Build history of the part. All positions in model axes, mm. A direction names the side the tool comes from. Give positions to 0.01 mm unless a question says otherwise; leave off trailing zeros. Order: outer loops, then holes, each group sorted by start corner. A loop starts at its lowest first (then second) coordinate and runs counter-clockwise, first axis right, second up. Notation, with made-up numbers: (-4, 19.5) -> (40, 19.5) arc R7 cw to (40, 25.5) -> close; hole circle Ø3 at (31, 7.25). An arc over 180 degrees is marked (long way). One line per question, with ' | ' between items. Start each with the question number.
(1) Cut at A-A (y = 241). Give the number of separate pieces and of enclosed holes in the cut face, then the cut area to 3 significant figures.
(2) Pin check, flat tips, straight feed: pin 1 Ø9.5 at (y, z) = (290, 16.5) entering from +X; pin 2 Ø2 at (x, y) = (-1077, -46) entering from +Z; pin 3 Ø9.5 at (x, z) = (-1638, 15) entering from +Y; pin 4 Ø2 at (y, z) = (271, 33.5) entering from +X. Stop position of each tip, or through.
(3) Which spindle directions (+Z, -Z, +X, -X, +Y, -Y) get a long thin tool onto all of the face, cutting with end or side? Do faces 1 (the face through (-2160.586, -325, 25)), 2 (the face through (0, 109, 25)), 3 (the face through (-1174, 155, 31.75)). Say none if no direction does.
(4) Cut at D-D (x = -989). Give the cut face in (y, z), then the cut area to 3 significant figures.
(5) Cut at B-B (x = -1476). Give the cut face in (y, z), then the cut area to 3 significant figures.
(6) Pull direction Y, two halves, no side cores. Call faces 4 (the face through (-1098, -116, 0)), 5 (the face through (-1163, 138.261, 38)), 6 (the face through (-1009, -296.136, 38)), 7 (the face through (-1097, -197, 31.75)): +Y half, -Y half, draft (parallel to the pull), parting line (faces both ways), or undercut.
(7) Drill centre lines: L1, parallel to Y at x = -1071, z = 34.5; L2, parallel to X at y = -323.5, z = 31 (3 decimals); L3, parallel to Y at x = -1812, z = 10. Where is each one in solid material? Low to high. Write a range as from..to.
from build123d import *

# Parameters (mm, degrees)
F2_DEPTH = 31.75
F1_W     = 2314.862013
F1_H     = 57.149999
F1_W_2   = 2314.703077
F1_H_2   = 57.15
F3_DEPTH = 50.8


with BuildPart() as f2:
    # F0 (on Top) → F2 (new body)
    with BuildSketch(Plane.XY):
        with BuildLine():
            Line((141.605, 0), (0, 0))
            Line((0, 0), (-0.017486, 172.135651))
            Line((-0.017486, 172.135651), (-0.017486, 400.964946))
            Line((-0.017486, 400.964946), (-154.322486, 400.964946))
            Line((-154.322486, 400.964946), (-154.322486, 172.135651))
            Line((-154.322486, 172.135651), (-308.627486, 172.135651))
            Line((-308.627486, 172.135651), (-308.627486, 400.964946))
            Line((-308.627486, 400.964946), (-462.932486, 400.964946))
            Line((-462.932486, 400.964946), (-462.932486, 172.135651))
            Line((-462.932486, 172.135651), (-617.237486, 172.135651))
            Line((-617.237486, 172.135651), (-617.237486, 400.964946))
            Line((-617.237486, 400.964946), (-771.542486, 400.964946))
            Line((-771.542486, 400.964946), (-771.542486, 172.135651))
            Line((-771.542486, 172.135651), (-925.847486, 172.135651))
            Line((-925.847486, 172.135651), (-925.847486, 400.964946))
            Line((-925.847486, 400.964946), (-1080.152486, 400.964946))
            Line((-1080.152486, 400.964946), (-1080.152486, 172.135651))
            Line((-1080.152486, 172.135651), (-1234.457486, 172.135651))
            Line((-1234.457486, 172.135651), (-1234.457486, 400.964946))
            Line((-1234.457486, 400.964946), (-1388.762486, 400.964946))
            Line((-1388.762486, 400.964946), (-1388.762486, 172.135651))
            Line((-1388.762486, 172.135651), (-1543.067486, 172.135651))
            Line((-1543.067486, 172.135651), (-1543.067486, 399.883687))
            Line((-1543.067486, 399.883687), (-1697.372486, 399.883687))
            Line((-1697.372486, 399.883687), (-1697.372486, 172.135651))
            Line((-1697.372486, 172.135651), (-1851.677486, 172.135651))
            Line((-1851.677486, 172.135651), (-1851.677486, 399.883687))
            Line((-1851.677486, 399.883687), (-2005.982486, 399.883687))
            Line((-2005.982486, 399.883687), (-2005.982486, 172.135651))
            Line((-2005.982486, 172.135651), (-2160.287486, 172.135651))
            Line((-2160.287486, 172.135651), (-2160.287486, 399.883687))
            Line((-2160.287486, 399.883687), (-2314.592486, 399.883687))
            Line((-2314.592486, 399.883687), (-2314.592486, 0))
            Line((-2314.592486, 0), (-2172.987486, 0))
            ThreePointArc((-2172.987486, 0), (-2164.00723, -3.719744), (-2160.287486, -12.7))
            Line((-2160.287486, -12.7), (-2160.287486, -97.307886))
            ThreePointArc((-2160.287486, -97.307886), (-2164.00723, -106.288142), (-2172.987486, -110.007886))
            Line((-2172.987486, -110.007886), (-2301.892486, -110.007886))
            ThreePointArc((-2301.892486, -110.007886), (-2310.872742, -113.72763), (-2314.592486, -122.707886))
            Line((-2314.592486, -122.707886), (-2314.592486, -207.315286))
            ThreePointArc((-2314.592486, -207.315286), (-2310.872742, -216.295542), (-2301.892486, -220.015286))
            Line((-2301.892486, -220.015286), (-2160.287486, -220.015286))
            Line((-2160.287486, -220.015286), (-2160.287486, -647.870064))
            Line((-2160.287486, -647.870064), (-2005.973684, -647.870064))
            Line((-2005.973684, -647.870064), (-2005.973684, -389.817446))
            Line((-2005.973684, -389.817446), (-1851.668684, -389.817446))
            Line((-1851.668684, -389.817446), (-1851.668684, -647.870064))
            Line((-1851.668684, -647.870064), (-1697.355, -647.870064))
            Line((-1697.355, -647.870064), (-1697.355, -389.817446))
            Line((-1697.355, -389.817446), (-1543.05, -389.817446))
            Line((-1543.05, -389.817446), (-1543.05, -647.870064))
            Line((-1543.05, -647.870064), (-1388.745, -647.870064))
            Line((-1388.745, -647.870064), (-1388.745, -389.817446))
            Line((-1388.745, -389.817446), (-1234.44, -389.817446))
            Line((-1234.44, -389.817446), (-1234.44, -647.870064))
            Line((-1234.44, -647.870064), (-1080.135, -647.870064))
            Line((-1080.135, -647.870064), (-1080.135, -389.817446))
            Line((-1080.135, -389.817446), (-925.83, -389.817446))
            Line((-925.83, -389.817446), (-925.83, -647.870064))
            Line((-925.83, -647.870064), (-771.525, -647.870064))
            Line((-771.525, -647.870064), (-771.525, -389.817446))
            Line((-771.525, -389.817446), (-617.22, -389.817446))
            Line((-617.22, -389.817446), (-617.22, -647.870064))
            Line((-617.22, -647.870064), (-462.915, -647.870064))
            Line((-462.915, -647.870064), (-462.915, -389.817446))
            Line((-462.915, -389.817446), (-308.61, -389.817446))
            Line((-308.61, -389.817446), (-308.61, -647.870064))
            Line((-308.61, -647.870064), (-154.305, -647.870064))
            Line((-154.305, -647.870064), (-154.305, -389.817446))
            Line((-154.305, -389.817446), (0, -389.817446))
            Line((0, -389.817446), (0, -647.870064))
            Line((0, -647.870064), (154.305, -647.870064))
            Line((154.305, -647.870064), (154.305, -220.015286))
            Line((154.305, -220.015286), (12.7, -220.015286))
            ThreePointArc((12.7, -220.015286), (3.719744, -216.295542), (0, -207.315286))
            Line((0, -207.315286), (0, -122.707886))
            ThreePointArc((0, -122.707886), (3.719744, -113.72763), (12.7, -110.007886))
            Line((12.7, -110.007886), (141.605, -110.007886))
            ThreePointArc((141.605, -110.007886), (150.585256, -106.288142), (154.305, -97.307886))
            Line((154.305, -97.307886), (154.305, -12.7))
            ThreePointArc((154.305, -12.7), (150.585256, -3.719744), (141.605, 0))
        make_face()
    extrude(amount=F2_DEPTH)

    # F1 (on face) → F3 (join)
    with BuildSketch(Plane.XY):
        with Locations((-1157.431006, 109.685767)):
            Rectangle(F1_W, F1_H)
        with Locations((-1003.234818, -324.710694)):
            Rectangle(F1_W_2, F1_H_2)
    extrude(amount=F3_DEPTH)


solid = f2.part
Result set:
1) separate pieces: 8 | enclosed holes: 0 | area: 39,200 mm2
2) pin 1: stops at x = -0.02 | pin 2: stops at z = 31.75 | pin 3: stops at y = 399.88 | pin 4: passes through
3) face 1: +Z, -Z, -X, -Y | face 2: +Z, -Z, +X, +Y | face 3: +Z, +X, -X, +Y
4) outline: (-389.82, 0) -> (400.96, 0) -> (400.96, 31.75) -> (138.26, 31.75) -> (138.26, 50.8) -> (81.11, 50.8) -> (81.11, 31.75) -> (-296.14, 31.75) -> (-296.14, 50.8) -> (-353.29, 50.8) -> (-353.29, 31.75) -> (-389.82, 31.75) -> close | area: 27,300 mm2
5) outline: (-647.87, 0) -> (172.14, 0) -> (172.14, 31.75) -> (138.26, 31.75) -> (138.26, 50.8) -> (81.11, 50.8) -> (81.11, 31.75) -> (-296.14, 31.75) -> (-296.14, 50.8) -> (-353.29, 50.8) -> (-353.29, 31.75) -> (-647.87, 31.75) -> close | area: 28,200 mm2
6) face 4: draft | face 5: +Y half | face 6: undercut | face 7: undercut
7) L1: y = -353.29..-296.14, 81.11..138.26 | L2: x = -2160.586..154.305 | L3: y = -647.87..172.14
